Here's how the part is built. I have some questions about the finished solid (model axes, mm). Face numbers are marked on the shaded views. A direction names the side the tool comes from. Round coordinates to 2 decimals unless told otherwise and drop trailing zeros. Write each loop counter-clockwise with the first axis right and the second up, starting at its lowest first coordinate (ties: lowest second). Pieces come first, ordered by that corner, then holes. Notation, with made-up numbers: (48.5, 15) - (70.5, 15) arc R25 cw to (70.5, 38) - close; hole circle Ø11 at (3, 6.25). An arc over 180 degrees is marked (long way). Use one line per item in the form item = value. Start each with the question number.
1. We'd pull the mould along X, two halves only. Please class the marked faces 6, 7, 8 and 9: +X half, -X half, draft (parallel to the pull), parting line (faces both ways), or undercut.
2. Which directions (+Z, -Z, +X, -X, +Y, -Y) give clear straight access to the entire face, cutting with the end or side of a thin tool? Please do the marked faces 1, 2, 3, 4 and 5.
3. I want a section at A-A, the plane x = 0. List the corners of the cut face in (y, z) for me, plus the area to 3 significant figures.
4. I want a section at B-B, the plane z = 0. List the corners of the cut face in (x, y) for me.
5. I want a section at D-D, the plane x = -25. List the corners of the cut face in (y, z) for me.
6. Will these pins go through, and if not, where does the flat tip stop? pin 1 (8 mm diameter, centred on x = 46, y = 4, fed in from -Z); pin 2 (1.2 mm diameter, centred on x = -7.5, y = 2.5, fed in from -Z); pin 3 (1.6 mm diameter, centred on y = 23.5, z = -39.5, fed in from -X); pin 4 (2 mm diameter, centred on x = 2, z = -39.5, fed in from +Y).
7. If I drill on line 1 along X through (y, z) = (17.5, 0); line 2 along Z through (x, y) = (-1.5, 6); line 3 along Z through (x, y) = (90, 0.7), over which ranges is the centre line in solid material (lowest first)?
8. I want a section at C-C, the plane z = 20. List the corners of the cut face in (x, y) for me.
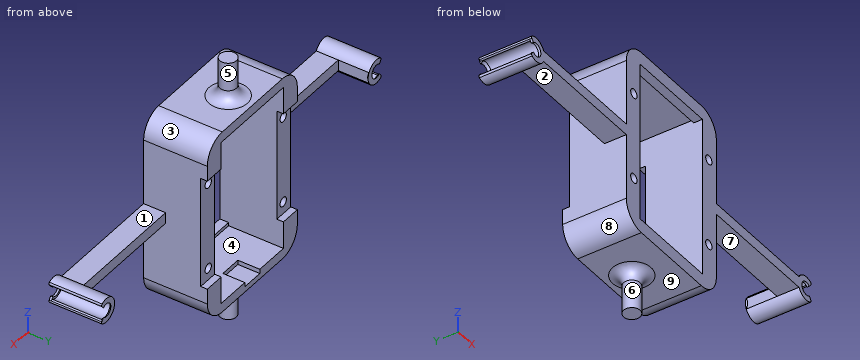
```python
from build123d import *

# Parameters (mm, degrees)
BOSS_EXTRUDE1_DEPTH  = 24
SKETCH22_W           = 60.00000000000001
SKETCH22_H           = 85
BOSS_EXTRUDE6_DEPTH  = 5
SKETCH5_W            = 41.5
SKETCH5_H            = 76
CUT_EXTRUDE1_DEPTH   = 25
SKETCH17_W           = 60
SKETCH17_H           = 51
CUT_EXTRUDE10_DEPTH  = 3
SKETCH8_W            = 55.101020514433614
SKETCH8_H            = 14
CUT_EXTRUDE3_DEPTH   = 108.77225201740228
FILLET4_R            = 10
BOSS_EXTRUDE3_DEPTH  = 1
BOSS_EXTRUDE3_DRAFT  = -45.0000000000001
MIRROR6_COPY_1_DEPTH = 1
MIRROR6_COPY_1_DRAFT = -45.0000000000001
BOSS_EXTRUDE4_DEPTH  = 1
FILLET3_R            = 0.75
SKETCH15_R           = 2.100000000000001
CUT_EXTRUDE8_DEPTH   = 106.67266341818518
SKETCH20_W           = 41.499999999999986
SKETCH20_H           = 72.99999999999999
CUT_EXTRUDE11_DEPTH  = 5
SKETCH21_R           = 3.75
BOSS_EXTRUDE5_DEPTH  = 18
FILLET5_R            = 5
SKETCH24_W           = 10
SKETCH24_H           = 2
CUT_EXTRUDE12_DEPTH  = 10


with BuildPart() as part:
    # Sketch4 → Boss-Extrude1 (new body)
    with BuildSketch(Plane(origin=(0, 0, 0), x_dir=(1, 0, 0), z_dir=(0, 1, 0))):
        with BuildLine():
            Line((-30, 2.499999999999996), (-30, 42.5))
            Line((-30, 42.5), (30, 42.5))
            Line((30, 42.5), (30, 2.499999999999996))
            Line((30, 2.499999999999996), (85.10102051443361, 2.49999999999999))
            ThreePointArc((85.10102051443361, 2.49999999999999), (88.90515510613471, 5.389927147780134), (93.53533185327602, 4.213244437154374))
            Line((93.53533185327602, 4.213244437154374), (92.57115043874622, 3.064177772475905))
            ThreePointArc((92.57115043874622, 3.064177772475905), (86, -2.572e-14), (92.57115043874622, -3.0641777724758823))
            Line((92.57115043874622, -3.0641777724758823), (93.53533185327602, -4.213244437154351))
            ThreePointArc((93.53533185327602, -4.213244437154351), (88.90515510613471, -5.389927147780135), (85.10102051443361, -2.499999999999969))
            Line((85.10102051443361, -2.499999999999969), (30, -2.4999999999999893))
            Line((30, -2.4999999999999893), (30.00000000000001, -42.499999999999986))
            Line((30.00000000000001, -42.499999999999986), (-30.00000000000001, -42.499999999999986))
            Line((-30.00000000000001, -42.499999999999986), (-30, -2.4999999999999893))
            Line((-30, -2.4999999999999893), (-85.10102051443361, -2.499999999999969))
            ThreePointArc((-85.10102051443361, -2.499999999999969), (-88.90515510613471, -5.389927147780135), (-93.53533185327602, -4.213244437154351))
            Line((-93.53533185327602, -4.213244437154351), (-92.57115043874622, -3.0641777724758823))
            ThreePointArc((-92.57115043874622, -3.0641777724758823), (-86, -2.523e-14), (-92.57115043874622, 3.064177772475905))
            Line((-92.57115043874622, 3.064177772475905), (-93.53533185327602, 4.213244437154374))
            ThreePointArc((-93.53533185327602, 4.213244437154374), (-88.90515510613471, 5.389927147780134), (-85.10102051443361, 2.49999999999999))
            Line((-85.10102051443361, 2.49999999999999), (-30, 2.499999999999996))
        make_face()
    extrude(amount=BOSS_EXTRUDE1_DEPTH)

    # Sketch22 → Boss-Extrude6 (add)
    with BuildSketch(Plane(origin=(0, 24, 0), x_dir=(1, 0, 0), z_dir=(0, 1, 0))):
        Rectangle(SKETCH22_W, SKETCH22_H)
    extrude(amount=BOSS_EXTRUDE6_DEPTH)

    # Sketch5 → Cut-Extrude1 (cut)
    with BuildSketch(Plane(origin=(0, 29, 0), x_dir=(1, 0, 0), z_dir=(0, 1, 0))):
        Rectangle(SKETCH5_W, SKETCH5_H)
    extrude(amount=-CUT_EXTRUDE1_DEPTH, mode=Mode.SUBTRACT)

    # Sketch17 → Cut-Extrude10 (cut)
    with BuildSketch(Plane(origin=(0, 29, 0), x_dir=(1, 0, 0), z_dir=(0, 1, 0))):
        Rectangle(SKETCH17_W, SKETCH17_H)
    extrude(amount=-CUT_EXTRUDE10_DEPTH, mode=Mode.SUBTRACT)

    # Sketch8 → Cut-Extrude3 (cut, through all)
    with BuildSketch(Plane.XY.offset(2.5000000000000004)):
        with Locations((-57.55051025721681, 17)):
            Rectangle(SKETCH8_W, SKETCH8_H)
        with Locations((57.55051025721681, 17)):
            Rectangle(SKETCH8_W, SKETCH8_H)
    extrude(amount=-CUT_EXTRUDE3_DEPTH, mode=Mode.SUBTRACT)

    # Fillet4
    fillet4_edges = [part.edges().sort_by_distance(p)[0] for p in [
        (-30, 14.5, -42.5),
        (30, 14.5, -42.5),
        (30.000000000000007, 14.5, 42.49999999999999),
        (-30.000000000000007, 14.5, 42.49999999999999),
    ]]
    fillet(fillet4_edges, radius=FILLET4_R)


with BuildPart() as boss_extrude3_tool:
    # Sketch11 → Boss-Extrude3 (with draft: the straight prism first)
    with BuildSketch(Plane(origin=(0, 24, 0), x_dir=(1, 0, 0), z_dir=(0, 1, 0))):
        with BuildLine():
            Line((-93.535331853276, 4.21324443715433), (-91.92836282905964, 2.2981333293569084))
            ThreePointArc((-91.92836282905964, 2.2981333293569084), (-87.00000000000001, -1.768e-14), (-91.92836282905964, -2.2981333293569084))
            Line((-91.92836282905964, -2.2981333293569084), (-93.535331853276, -4.21324443715433))
            ThreePointArc((-93.535331853276, -4.21324443715433), (-84.50000000000001, -1.835e-14), (-93.535331853276, 4.21324443715433))
        make_face()
    extrude(amount=-BOSS_EXTRUDE3_DEPTH)
    # Boss-Extrude3: the draft: its side faces are tilted about the plane it starts from
    boss_extrude3_sides = [boss_extrude3_tool.faces().sort_by_distance(p)[0] for p in [
        (-92.731847341, 23.5, -3.255688883),
        (-87, 23.5, 0),
        (-92.731847341, 23.5, 3.255688883),
        (-84.5, 23.5, 0),
    ]]
    draft(boss_extrude3_sides, Plane(origin=(0, 24, 0), x_dir=(1, 0, 0), z_dir=(0, 1, 0)), BOSS_EXTRUDE3_DRAFT)


with BuildPart() as part_1:
    add(part.part)

    # Boss-Extrude3: add boss_extrude3_tool
    add(boss_extrude3_tool.part)


with BuildPart() as mirror6_copy_1_tool:
    # Mirror6 copy 1 sketch → Mirror6 copy 1 (with draft: the straight prism first)
    with BuildSketch(Plane(origin=(0, 24, 0), x_dir=(-1, 0, 0), z_dir=(0, 1, 0))):
        with BuildLine():
            Line((-93.535331853276, -4.21324443715433), (-91.92836282905964, -2.2981333293569084))
            ThreePointArc((-91.92836282905964, -2.2981333293569084), (-87.00000000000001, 1.768e-14), (-91.92836282905964, 2.2981333293569084))
            Line((-91.92836282905964, 2.2981333293569084), (-93.535331853276, 4.21324443715433))
            ThreePointArc((-93.535331853276, 4.21324443715433), (-84.50000000000001, 1.835e-14), (-93.535331853276, -4.21324443715433))
        make_face()
    extrude(amount=-MIRROR6_COPY_1_DEPTH)
    # Mirror6 copy 1: the draft: its side faces are tilted about the plane it starts from
    mirror6_copy_1_sides = [mirror6_copy_1_tool.faces().sort_by_distance(p)[0] for p in [
        (92.731847341, 23.5, -3.255688883),
        (87, 23.5, 0),
        (92.731847341, 23.5, 3.255688883),
        (84.5, 23.5, 0),
    ]]
    draft(mirror6_copy_1_sides, Plane(origin=(0, 24, 0), x_dir=(-1, 0, 0), z_dir=(0, 1, 0)), MIRROR6_COPY_1_DRAFT)


with BuildPart() as part_2:
    add(part_1.part)

    # Mirror6 copy 1: add mirror6_copy_1_tool
    add(mirror6_copy_1_tool.part)

    # Sketch12 → Boss-Extrude4 (add)
    with BuildSketch(Plane.XZ):
        with BuildLine():
            Line((-93.53533185327602, 4.213244437154351), (-91.92836282905965, 2.2981333293569315))
            ThreePointArc((-91.92836282905965, 2.2981333293569315), (-87, 1.768e-14), (-91.92836282905964, -2.298133329356913))
            Line((-91.92836282905964, -2.298133329356913), (-93.53533185327602, -4.213244437154374))
            ThreePointArc((-93.53533185327602, -4.213244437154374), (-84.49999999999996, 2.568e-14), (-93.53533185327602, 4.213244437154351))
        make_face()
    boss_extrude4 = extrude(amount=-BOSS_EXTRUDE4_DEPTH)

    # Mirror5: Boss-Extrude4 across plane
    add(boss_extrude4.mirror(Plane(origin=(0, 0, 0), x_dir=(0, 0, 1), z_dir=(1, 0, 0))))

    # Fillet3
    fillet3_edges = [part_2.edges().sort_by_distance(p)[0] for p in [
        (93.535331853276, 12, 4.213244437154348),
        (92.57115043874622, 12.5, 3.064177772475879),
        (92.57115043874622, 12.5, -3.064177772475902),
        (93.535331853276, 12, -4.213244437154364),
        (-93.535331853276, 12, 4.213244437154348),
        (-92.57115043874622, 12.5, 3.064177772475879),
        (-93.535331853276, 12, -4.213244437154364),
        (-92.57115043874622, 12.5, -3.064177772475902),
    ]]
    fillet(fillet3_edges, radius=FILLET3_R - 0.0001)  # a hair under: the kernel refuses the full size

    # Sketch15 → Cut-Extrude8 (cut, through all)
    with BuildSketch(Plane(origin=(0, 26.000000000000004, 0), x_dir=(1, 0, 0), z_dir=(0, 1, 0))):
        with Locations(Location((-25, 20.000000000000004, 0), (0, 0, 270))):
            Circle(SKETCH15_R)
        with Locations(Location((25, 20.000000000000004, 0), (0, 0, 90))):
            Circle(SKETCH15_R)
        with Locations(Location((25, -20.000000000000004, 0), (0, 0, 270))):
            Circle(SKETCH15_R)
        with Locations(Location((-25, -20.000000000000004, 0), (0, 0, 90))):
            Circle(SKETCH15_R)
    extrude(amount=-CUT_EXTRUDE8_DEPTH, mode=Mode.SUBTRACT)

    # Sketch20 → Cut-Extrude11 (cut)
    with BuildSketch(Plane(origin=(0, 4, 0), x_dir=(1, 0, 0), z_dir=(0, 1, 0))):
        Rectangle(SKETCH20_W, SKETCH20_H)
    extrude(amount=-CUT_EXTRUDE11_DEPTH, mode=Mode.SUBTRACT)

    # Sketch21 → Boss-Extrude5 (add)
    with BuildSketch(Plane.XY.offset(42.499999999999986)):
        with Locations(Location((0, 18, 0), (0, 0, 180))):
            Circle(SKETCH21_R)
    boss_extrude5 = extrude(amount=BOSS_EXTRUDE5_DEPTH)

    # Mirror9: Boss-Extrude5 across plane
    add(boss_extrude5.mirror(Plane.XY))

    # Fillet5
    fillet5_edges = [part_2.edges().sort_by_distance(p)[0] for p in [
        (3.75, 17.999999999999996, 42.499999999999986),
        (3.75, 17.999999999999996, -42.499999999999986),
    ]]
    fillet(fillet5_edges, radius=FILLET5_R)

    # Sketch24 → Cut-Extrude12 (cut)
    with BuildSketch(Plane(origin=(0, 29, 0), x_dir=(1, 0, 0), z_dir=(0, 1, 0))):
        with Locations((0, 38.999999999999986)):
            Rectangle(SKETCH24_W, SKETCH24_H)
    extrude(amount=-CUT_EXTRUDE12_DEPTH, mode=Mode.SUBTRACT)


solid = part_2.part
```
Model answer:
q1.face_6 = parting line
q1.face_7 = undercut
q1.face_8 = -X half
q1.face_9 = draft
q2.face_1 = +Z, +Y, -Y
q2.face_2 = -Z, +Y, -Y
q2.face_3 = +Z, +X, +Y, -Y
q2.face_4 = +Y
q2.face_5 = +Z
q3.outline = (0, -42.5) - (9.25, -42.5) arc R5 cw to (14.25, -47.5) - (14.25, -60.5) - (21.75, -60.5) - (21.75, -47.5) arc R5 cw to (26.75, -42.5) - (29, -42.5) - (29, -40) - (19, -40) - (19, -38) - (4, -38) - (4, -36.5) - (0, -36.5) - close; (0, 36.5) - (4, 36.5) - (4, 38) - (29, 38) - (29, 42.5) - (26.75, 42.5) arc R5 cw to (21.75, 47.5) - (21.75, 60.5) - (14.25, 60.5) - (14.25, 47.5) arc R5 cw to (9.25, 42.5) - (0, 42.5) - close
q3.area = 544 mm2
q4.outline = (-87, 0) - (-20.75, 0) - (-20.75, 26) - (-30, 26) - (-30, 10) - (-85.1, 10) - (-85.1, 23.4) - (-84.5, 24) - (-87, 24) - (-86, 23) - (-86, 1) - (-87, 1) - close; (20.75, 0) - (87, 0) - (87, 1) - (86, 1) - (86, 23) - (87, 24) - (84.5, 24) - (85.1, 23.4) - (85.1, 10) - (30, 10) - (30, 26) - (20.75, 26) - close
q5.outline = (0, -41.16) - (29, -41.16) - (29, -25.5) - (26, -25.5) - (26, -22.1) - (0, -22.1) - close; (0, -17.9) - (26, -17.9) - (26, 17.9) - (0, 17.9) - close; (0, 22.1) - (26, 22.1) - (26, 25.5) - (29, 25.5) - (29, 41.16) - (0, 41.16) - close
q6.pin_1 = -2.5
q6.pin_2 = -42.5
q6.pin_3 = -27.85
q6.pin_4 = 29
q7.line_1 = -86 to -85.1, -30 to -20.75, 20.75 to 30, 85.1 to 86
q7.line_2 = -42.5 to -38, 38 to 42.5
q7.line_3 = -5.5 to -3, 3 to 5.5
q8.outline = (-30, 0) - (-27.1, 0) - (-27.1, 26) - (-30, 26) - close; (-22.9, 0) - (-20.75, 0) - (-20.75, 26) - (-22.9, 26) - close; (20.75, 0) - (22.9, 0) - (22.9, 26) - (20.75, 26) - close; (27.1, 0) - (30, 0) - (30, 26) - (27.1, 26) - close
